Model file for the job. Use its own axes, mm. A direction names the side the tool comes from. Round coordinates to 2 decimals unless told otherwise and drop trailing zeros. Loops run counter-clockwise (first coordinate to the right, second up) from the corner with the lowest first, then second, coordinate; pieces in that order, holes last.
from build123d import *

# Parameters (mm, degrees)
F0_R      = 50.8
F1_DEPTH  = 3.175
F2_R      = 50.8
F3_DEPTH  = 3.175
F4_R      = 44.45
F5_DEPTH  = 3.175
F6_R      = 38.1
F7_DEPTH  = 3.175
F8_R      = 31.75
F9_DEPTH  = 3.175
F10_R     = 25.4
F11_DEPTH = 3.175
F12_R     = 19.05
F13_DEPTH = 3.175
F14_R     = 11.43
F15_DEPTH = 22.225


with BuildPart() as f1:
    # F0 (on Front) → F1 (new body)
    with BuildSketch(Plane.XZ):
        Circle(F0_R)
    extrude(amount=F1_DEPTH)

    # F2 (on face) → F3 (join)
    with BuildSketch(Plane.XZ.offset(3.175)):
        Circle(F2_R)
    extrude(amount=F3_DEPTH)

    # F4 (on face) → F5 (join)
    with BuildSketch(Plane.XZ.offset(6.35)):
        Circle(F4_R)
    extrude(amount=F5_DEPTH)

    # F6 (on face) → F7 (join)
    with BuildSketch(Plane.XZ.offset(9.525)):
        Circle(F6_R)
    extrude(amount=F7_DEPTH)

    # F8 (on face) → F9 (join)
    with BuildSketch(Plane.XZ.offset(12.7)):
        Circle(F8_R)
    extrude(amount=F9_DEPTH)

    # F10 (on face) → F11 (join)
    with BuildSketch(Plane.XZ.offset(15.875)):
        Circle(F10_R)
    extrude(amount=F11_DEPTH)

    # F12 (on face) → F13 (join)
    with BuildSketch(Plane.XZ.offset(19.05)):
        Circle(F12_R)
    extrude(amount=F13_DEPTH)

    # F14 (on face) → F15 (cut)
    with BuildSketch(Plane.XZ.offset(22.225)):
        Circle(F14_R)
    extrude(amount=-F15_DEPTH, mode=Mode.SUBTRACT)


solid = f1.part
Q1. Flat gauge pins, fed straight in: P1, Ø4, axis at y = -20, z = 20, coming from the +X side; P2, Ø1.5, axis at x = -9.5, z = 1, coming from the -Y side; P3, Ø3, axis at y = -6, z = 22.5, coming from the -X side; P4, Ø12, axis at y = -4.5, z = -28, coming from the +X side. Where does each tip first touch, or does it go through?
Q2. Pull direction X, two halves, no side cores. Call faces 1 (the face through (-1, 0, 12)), 2 (the face through (10.902, -11.268, 3.433)), 3 (the face through (-5.506, -17.44, -24.796)): pulls with the +X half, pulls with the -X half, needs draft (parallel to the pull), parting line crosses it, or undercut.
Q3. Slice it at D-D on x = 35.5. Give the cut face in (y, z) (3 decimals), plus the area to 3 significant figures.
Q4. Slice it at C-C on y = -20.5. Give the cut face in (x, z), plus the area to 3 significant figures.
Q5. Slice it at A-A on x = 0. Give the cut face in (y, z) (3 decimals), plus the area to 3 significant figures.
Q6. Tool access for faces 4 (the face through (-6.883, -14.265, -30.995)), 5 (the face through (8.2, -22.225, -8.2)): list every direction of +Z, -Z, +X, -X, +Y, -Y with a clear straight run to the whole face (end or side of a thin tool).
Q7. Slice it at B-B on z = 0. Give the cut face in (x, y) (3 decimals), plus the area to 3 significant figures.
Q8. Probe line 1 (X direction, y = -7.5, z = -0.5); line 2 (Z direction, x = 0, y = -8.75); line 3 (Z direction, x = 0, y = -13). List the from-to ranges inside material, lowest first.
Reply:
1. P1: stops at x = 17.68
1. P2: passes through
1. P3: stops at x = -46.26
1. P4: stops at x = 45.79
2. face 1: needs draft
2. face 2: undercut
2. face 3: parting line crosses it
3. outline: (-12.7, -13.833) - (-9.525, -13.833) - (-9.525, -26.75) - (-6.35, -26.75) - (-6.35, -36.337) - (0, -36.337) - (0, 36.337) - (-6.35, 36.337) - (-6.35, 26.75) - (-9.525, 26.75) - (-9.525, 13.833) - (-12.7, 13.833) - close
3. area: 719 mm2
4. outline: circle Ø38.1 at (0, 0); hole circle Ø22.86 at (0, 0)
4. area: 730 mm2
5. outline: (-22.225, -19.05) - (-19.05, -19.05) - (-19.05, -25.4) - (-15.875, -25.4) - (-15.875, -31.75) - (-12.7, -31.75) - (-12.7, -38.1) - (-9.525, -38.1) - (-9.525, -44.45) - (-6.35, -44.45) - (-6.35, -50.8) - (0, -50.8) - (0, -11.43) - (-22.225, -11.43) - close; (-22.225, 11.43) - (0, 11.43) - (0, 50.8) - (-6.35, 50.8) - (-6.35, 44.45) - (-9.525, 44.45) - (-9.525, 38.1) - (-12.7, 38.1) - (-12.7, 31.75) - (-15.875, 31.75) - (-15.875, 25.4) - (-19.05, 25.4) - (-19.05, 19.05) - (-22.225, 19.05) - close
5. area: 1,150 mm2
6. face 4: -Y
6. face 5: +Z, -Z, +X, -X, -Y
7. outline: (-50.8, -6.35) - (-44.45, -6.35) - (-44.45, -9.525) - (-38.1, -9.525) - (-38.1, -12.7) - (-31.75, -12.7) - (-31.75, -15.875) - (-25.4, -15.875) - (-25.4, -19.05) - (-19.05, -19.05) - (-19.05, -22.225) - (-11.43, -22.225) - (-11.43, 0) - (-50.8, 0) - close; (11.43, -22.225) - (19.05, -22.225) - (19.05, -19.05) - (25.4, -19.05) - (25.4, -15.875) - (31.75, -15.875) - (31.75, -12.7) - (38.1, -12.7) - (38.1, -9.525) - (44.45, -9.525) - (44.45, -6.35) - (50.8, -6.35) - (50.8, 0) - (11.43, 0) - close
7. area: 1,150 mm2
8. line 1: x = -44.45 to -11.42, 11.42 to 44.45
8. line 2: z = -44.45 to -11.43, 11.43 to 44.45
8. line 3: z = -31.75 to -11.43, 11.43 to 31.75
